from build123d import *

# Parameters (mm, degrees)
F1_DEPTH  = 1.6
F2_R      = 3
F3_DEPTH  = 3
F6_R      = 0.5
F7_R      = 0.5
F8_R      = 0.5
F4_R      = 0.5
F9_DEPTH  = 4
F10_R     = 2.1
F11_DEPTH = 0.2


with BuildPart() as f1:
    # F0 (on Top) → F1 (new body)
    with BuildSketch(Plane.XY):
        with BuildLine():
            Line((70.716411, 29.285482), (6.37358, 29.285482))
            ThreePointArc((6.37358, 29.285482), (38.544995, 6.285482), (70.716411, 29.285482))
        make_face()
    extrude(amount=F1_DEPTH)

    # F2 (on face) → F3 (cut)
    with BuildSketch(Plane.XY.offset(1.6)):
        with Locations((14.544995, 23.785482)):
            Circle(F2_R)
        with Locations((62.544995, 23.785482)):
            Circle(F2_R)
    extrude(amount=-F3_DEPTH, mode=Mode.SUBTRACT)

    # F6 (on face) + F7 (on face) + F8 (on face) + F5 (on face) + F4 (on face) → F9 (cut)
    with BuildSketch(Plane.XY.offset(1.6)):
        with Locations((48.844995, 14.685482)):
            Circle(F6_R)
        with Locations((53.844995, 14.685482)):
            Circle(F6_R)
        with Locations((51.344995, 14.685482)):
            Circle(F6_R)
    with BuildSketch(Plane.XY.offset(1.6)):
        with Locations((37.294995, 26.285482)):
            Circle(F7_R)
        with Locations((39.794995, 26.285482)):
            Circle(F7_R)
    with BuildSketch(Plane.XY.offset(1.6)):
        with Locations((36.794995, 14.585482)):
            Circle(F8_R)
        with Locations((40.294995, 14.585482)):
            Circle(F8_R)
    with BuildSketch(Plane.XY.offset(1.6)):
        with BuildLine():
            ThreePointArc((51.044995, 23.185482), (50.794995, 22.935482), (51.044995, 22.685482))
            Line((51.044995, 22.685482), (52.044995, 22.685482))
            ThreePointArc((52.044995, 22.685482), (52.294995, 22.935482), (52.044995, 23.185482))
            Line((52.044995, 23.185482), (51.044995, 23.185482))
        make_face()
        with BuildLine():
            ThreePointArc((49.094995, 20.535482), (49.344995, 20.785482), (49.094995, 21.035482))
            Line((49.094995, 21.035482), (48.394995, 21.035482))
            ThreePointArc((48.394995, 21.035482), (48.144995, 20.785482), (48.394995, 20.535482))
            Line((48.394995, 20.535482), (49.094995, 20.535482))
        make_face()
        with BuildLine():
            Line((53.994995, 20.535482), (54.694995, 20.535482))
            ThreePointArc((54.694995, 20.535482), (54.944995, 20.785482), (54.694995, 21.035482))
            Line((54.694995, 21.035482), (53.994995, 21.035482))
            ThreePointArc((53.994995, 21.035482), (53.744995, 20.785482), (53.994995, 20.535482))
        make_face()
    with BuildSketch(Plane.XY.offset(1.6)):
        with Locations((24.544995, 21.285482)):
            Circle(F4_R)
        with Locations((26.544995, 21.285482)):
            Circle(F4_R)
        with Locations((28.544995, 21.285482)):
            Circle(F4_R)
    extrude(amount=-F9_DEPTH, mode=Mode.SUBTRACT)

    # F10 (on face) → F11 (cut)
    with BuildSketch(Plane(origin=(0, 0, 0), x_dir=(1, 0, 0), z_dir=(0, 0, -1))):
        with Locations((62.544995, -23.785482)):
            Circle(F10_R)
        with Locations((14.544995, -23.785482)):
            Circle(F10_R)
    extrude(amount=-F11_DEPTH, mode=Mode.SUBTRACT)


solid = f1.part
Geometry: final body of the model. Coordinates: model frame, mm. Coordinates: 2 decimals unless noted, no trailing zeros. Order: outer loops, then holes, each group sorted by start corner. A loop starts at its lowest first (then second) coordinate and runs counter-clockwise, first axis right, second up. Notation, with made-up numbers: (-12.5, 39.5) - (43.5, 39.5) arc R17 ccw to (43.5, 62.5) - close; hole circle Ø5 at (70, 4.5). An arc over 180 degrees is marked (long way). Use one line per item in the form item = value.
1) Pin query (flat end, axial travel): pin 1 (0.8 mm diameter, centred on x = 54.5, z = 1, fed in from -Y). Return the tip coordinate at first contact, or that it passes through.
Solutions:
pin_1 = 10.05
2) Section D-D (x = 64.5). Return loops of the section in (y, z).
Solutions:
outline = (18.32, 0) - (21.51, 0) - (21.51, 1.6) - (18.32, 1.6) - close; (26.06, 0) - (29.29, 0) - (29.29, 1.6) - (26.06, 1.6) - close
3) Section A-A (z = 1). State how many separate pieces and enclosed holes the cut face has, then the cut area to 3 significant figures.
Solutions:
separate_pieces = 1
enclosed_holes = 15
area = 1,010 mm^2
4) Ray query, L1, parallel to X at y = 26.5, z = 0.6; L2, parallel to X at y = 25.5, z = 0.85; L3, parallel to X at y = 24.5, z = 1.1. Return the intervals inside material, ascending.
Solutions:
L1 = 7.47 to 13.27, 15.82 to 36.84, 37.75 to 39.34, 40.25 to 61.27, 63.82 to 69.62
L2 = 7.93 to 12.08, 17.01 to 60.08, 65.01 to 69.16
L3 = 8.43 to 11.63, 17.46 to 59.63, 65.46 to 68.66
5) Section C-C (y = 19.5). Return loops of the section in (x, z), then the cut area to 3 significant figures.
Solutions:
outline = (11.64, 0) - (65.45, 0) - (65.45, 1.6) - (11.64, 1.6) - close
area = 86.1 mm^2
6) Section B-B (x = 16). Return loops of the section in (y, z).
Solutions:
outline = (14.84, 0) - (21.16, 0) - (21.16, 1.6) - (14.84, 1.6) - close; (26.41, 0) - (29.29, 0) - (29.29, 1.6) - (26.41, 1.6) - close
7) Mould query, pull axis X, two halves, no side actions, for faces 1 (the face through (38, 21, 0)), 2 (the face through (37.95, 6.29, 0.79)), 3 (the face through (17.406, 24.687, 0.811)). Classes: +X half, -X half, draft (parallel to the pull), parting line (faces both ways), or undercut.
Solutions:
face_1 = draft
face_2 = parting line
face_3 = undercut
